Autodesk Inventor part; units mm, degrees
ref_plane "YZ Plane" through (0, 0, 0) normal (1, 0, 0) x (0, 1, 0)
ref_plane "XZ Plane" through (0, 0, 0) normal (0, 1, 0) x (-1, 0, 0)
ref_plane "XY Plane" through (0, 0, 0) normal (0, 0, 1) x (1, 0, 0)
sketch "Sketch1" plane through (0, 0, 0) normal (0, 0, 1) x (1, 0, 0)
  circle A0 centre (0, 0) radius 8.5
  dimension "d0" = 17
extrude "Extrusion1" add sketch "Sketch1" along normal blind 75
sketch "Sketch2" plane through (0, 0, 0) normal (0, 1, 0) x (-1, 0, 0)
  circle A0 centre (0, 70) radius 1.5
  line L0 (8.5, 75) -> (-8.5, 75)
  circle A1 centre (0, 5) radius 1.5
  line L1 (8.5, 0) -> (-8.5, 0)
  point P0 (0, 0)
  dimension "d3" = 3
  dimension "d4" = 5
  dimension "d5" = 3
  dimension "d6" = 5
extrude "Extrusion2" cut sketch "Sketch2" against normal through all both and the other way through all
fillet "Fillet1" radius 2 2 edges at (-8.5, 0, 75) (-8.5, 0, 0)
sketch "Sketch5" plane through (0, 0, 75) normal (0, 0, 1) x (1, 0, 0)
  line L0 (-16.9, 6.5) -> (17, 6.5)
  line L1 (17, 6.5) -> (17, -6.5)
  line L2 (17, -6.5) -> (-16.9, -6.5)
  line L3 (-16.9, -6.5) -> (-16.9, 6.5)
  point P0 (0, 0)
  dimension "d18" = 13
  dimension "d19" = 6.5
extrude "Extrusion5" cut sketch "Sketch5" against normal blind 8
sketch "Sketch6" plane through (0, 0, 0) normal (0, 0, -1) x (-1, 0, 0)
  line L0 (-15.4684, 6.5) -> (16.538, 6.5)
  line L1 (16.538, 6.5) -> (16.538, -6.5)
  line L2 (16.538, -6.5) -> (-15.4684, -6.5)
  line L3 (-15.4684, -6.5) -> (-15.4684, 6.5)
  point P0 (0, 0)
  dimension "d22" = 13
  dimension "d23" = 6.5
extrude "Extrusion6" cut sketch "Sketch6" against normal blind 8
sketch "Sketch7" plane through (-5.4772, -6.5, 8) normal (0, 1, 0) x (1, 0, 0)
  circle A0 centre (5.4772, 3) radius 1.5
  line L0 (10.9545, -59) -> (0, -59)
  line L1 (0, -65) -> (0, -59)
  line L2 (10.9545, -59) -> (10.9545, -65)
  line L3 (10.9545, 0) -> (10.9545, -59)
  line L4 (0, 0) -> (10.9545, 0)
  line L5 (0, 0) -> (0, 6)
  line L6 (10.9545, 6) -> (10.9545, 0)
  line L7 (0, -59) -> (0, 0)
  circle A1 centre (5.4772, -62) radius 1.5
  point P0 (5.4772, 8)
  point P1 (5.4772, -67)
extrude "Extrusion7" add sketch "Sketch7" along normal blind 15 and the other way blind 2 contours A0
sketch "Sketch8" plane through (-5.4772, 6.5, 67) normal (0, -1, 0) x (1, 0, 0)
  circle A0 centre (5.4772, -62) radius 1.5
  line L0 (0, 0) -> (10.9545, 0)
  line L1 (10.9545, 6) -> (10.9545, 0)
  line L2 (0, 0) -> (0, 6)
  line L3 (0, -59) -> (0, 0)
  line L4 (10.9545, -59) -> (0, -59)
  line L5 (10.9545, -59) -> (10.9545, -65)
  line L6 (0, -65) -> (0, -59)
  line L7 (10.9545, 0) -> (10.9545, -59)
  circle A1 centre (5.4772, 3) radius 1.5
  point P0 (5.4772, -67)
  point P1 (5.4772, 8)
extrude "Extrusion8" add sketch "Sketch8" along normal blind 15 and the other way blind 2 contours A1
properties part number "cylinder right"
Verification items for the finished model (mm, model axes). A direction names the side the tool comes from. Give positions to 0.01 mm unless a question says otherwise; leave off trailing zeros. Loops run counter-clockwise (first coordinate to the right, second up) from the corner with the lowest first, then second, coordinate; pieces in that order, holes last.
1. Go/stop test with flat-tipped pins: pin 1 Ø3 at (x, y) = (-3.5, 4.5) entering from +Z; pin 2 Ø2 at (x, y) = (-2, -5) entering from +Z; pin 3 Ø6 at (x, y) = (6, -6) entering from -Z. Record where each tip stops, or that it passes through.
2. Section check B-B, the plane z = 5. Enter the section's corners in (x, y).
3. Set-up check for faces 1 (the flat face through (0, 8.5, 5)), 2 (the flat face through (0, 0, 8)): record each of +Z, -Z, +X, -X, +Y, -Y from which the full face is reachable in a straight line by a thin tool's end or side.
4. Thickness scan on line 1 (Y direction, x = 1.5, z = 68); line 2 (Z direction, x = -0.75, y = 2.5); line 3 (X direction, y = -0.5, z = 52.5). Record the ranges inside material, lowest first.
5. Mould release check, pull along Y, two halves, no side actions. Record for faces 3 (the flat face through (0, -8.5, 5)), 4 (the cylindrical face through (0.806, 0.091, 68.735)), 5 (the flat face through (0, 8.5, 70)): released by +Y, released by -Y, zero draft, split by the parting line, or undercut.
6. Section check A-A, the plane y = 1.5. Enter the section's corners in (x, z), then the cut area to 3 significant figures.
7. Section check C-C, the plane y = -5. Enter the section's corners in (x, z).
Geometry says:
1. pin 1: stops at z = 67
1. pin 2: stops at z = 71.12
1. pin 3: stops at z = 0.12
2. outline: (-5.48, -6.5) arc R8.5 ccw to (-1.5, -8.37) - (-1.5, -8.5) - (1.5, -8.5) - (1.5, -8.37) arc R8.5 ccw to (5.48, -6.5) - (1.5, -6.5) - (1.5, 6.5) - (5.48, 6.5) arc R8.5 ccw to (1.5, 8.37) - (1.5, 8.5) - (-1.5, 8.5) - (-1.5, 8.37) arc R8.5 ccw to (-5.48, 6.5) - (-1.5, 6.5) - (-1.5, -6.5) - close
3. face 1: +Z, -Z, +X, -X, +Y
3. face 2: +X, -X
4. line 1: y = -8.37 to -6.5, 6.5 to 8.37
4. line 2: z = 3.7 to 6.3, 8 to 67, 68.7 to 71.3
4. line 3: x = -8.49 to 8.49
5. face 3: released by -Y
5. face 4: undercut
5. face 5: released by +Y
6. outline: (-8.37, 8) - (8.37, 8) - (8.37, 67) - (-8.37, 67) - close; circle Ø3 at (0, 5); circle Ø3 at (0, 70)
6. area: 1,000 mm2
7. outline: (-6.87, 8) - (6.87, 8) - (6.87, 67) - (-6.87, 67) - close; circle Ø3 at (0, 5); circle Ø3 at (0, 70)
